Could you check a few things on this model? Use its own coordinates, in mm. Face numbers are marked on the shaded views. A direction names the side the tool comes from. Coordinates: 2 decimals unless noted, no trailing zeros. Loops run counter-clockwise (first coordinate to the right, second up) from the corner with the lowest first, then second, coordinate; pieces in that order, holes last. Notation, with made-up numbers: (-23.75, 7) -> (19.25, 7) arc R25 cw to (19.25, 42) -> close; hole circle Ø7 at (-10, 88). An arc over 180 degrees is marked (long way). One line per question, with ' | ' between items.
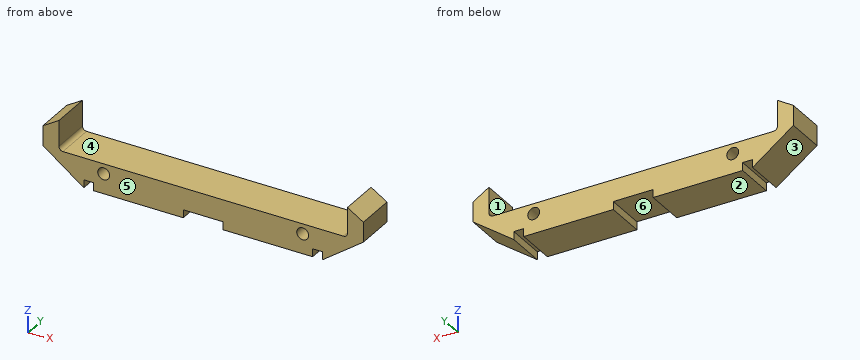
Autodesk Inventor part; units mm, degrees
ref_plane "YZ Plane" through (0, 0, 0) normal (1, 0, 0) x (0, 1, 0)
ref_plane "XZ Plane" through (0, 0, 0) normal (0, 1, 0) x (-1, 0, 0)
ref_plane "XY Plane" through (0, 0, 0) normal (0, 0, 1) x (1, 0, 0)
sketch "Esquisse1" plane through (0, 0, 0) normal (0, 1, 0) x (-1, 0, 0)
  circle A0 centre (0, 0) radius 25 construction
  line L0 (-25, 0) -> (25, 0) construction
  arc A1 (-75, -80.7775) -> (-75, 80.7775) centre (-25, 0) ccw construction
  arc A2 (75, 80.7775) -> (75, -80.7775) centre (25, 0) ccw construction
  line L1 (0, 25) -> (0, 0) construction
  line L2 (-75, 80.7775) -> (75, 80.7775)
  line L3 (-75, -80.7775) -> (75, -80.7775)
  arc A3 (75, -80.7775) -> (75, 80.7775) centre (25, 0) ccw
  arc A4 (-75, 80.7775) -> (-75, -80.7775) centre (-25, 0) ccw
  dimension "d0" = 50
  dimension "d1" = 190
  dimension "d2" = 150
extrude "Extrusion1" add sketch "Esquisse1" along normal mid plane 20
sketch "Esquisse4" plane through (0, -10, 0) normal (0, -1, 0) x (1, 0, 0)
  line L0 (-50, 40) -> (50, 40) construction
  line L1 (50, 40) -> (50, -40) construction
  line L2 (50, -40) -> (-50, -40) construction
  line L3 (-50, -40) -> (-50, 40) construction
  circle A0 centre (-50, 40) radius 3
  circle A1 centre (50, 40) radius 3
  circle A2 centre (50, -40) radius 3
  circle A3 centre (-50, -40) radius 3
  line L4 (75, 80.7775) -> (-75, 80.7775)
  point P0 (0, 0)
  dimension "d15" = 80
  dimension "d16" = 100
  dimension "d17" = 50
  dimension "d18" = 40
  dimension "d19" = 6
  dimension "d20" = 6
  dimension "d21" = 6
  dimension "d22" = 6
  dimension "d25" = 40.7775
extrude "Extrusion4" cut sketch "Esquisse4" against normal through all
sketch "Esquisse12" plane through (0, -10, 0) normal (0, -1, 0) x (1, 0, 0)
  circle A0 centre (50, -40) radius 3
  circle A1 centre (-50, 40) radius 3
  circle A2 centre (50, 40) radius 3
  circle A3 centre (-50, -40) radius 3
  line L0 (75, 80.7775) -> (-75, 80.7775)
  arc A4 (-75, 80.7775) -> (-75, -80.7775) centre (-25, 0) ccw
  line L1 (-75, -80.7775) -> (75, -80.7775)
  arc A5 (75, -80.7775) -> (75, 80.7775) centre (25, 0) ccw
  line L2 (-72.5, 60) -> (72.5, 60)
  line L3 (72.5, 60) -> (72.5, 45)
  line L4 (72.5, 45) -> (-72.5, 45)
  line L5 (-72.5, 45) -> (-72.5, 60)
  line L6 (-60, 45) -> (60, 45)
  line L7 (60, 45) -> (60, 30)
  line L8 (60, 30) -> (-60, 30)
  line L9 (-60, 30) -> (-60, 45)
  line L10 (-72.5, 45) -> (-80.5, 45)
  line L11 (-80.5, 45) -> (-80.5, 55)
  line L12 (-80.5, 55) -> (-72.5, 55)
  line L13 (-72.5, 55) -> (-72.5, 45)
  line L14 (72.5, 45) -> (80.5, 45)
  line L15 (80.5, 45) -> (80.5, 55)
  line L16 (80.5, 55) -> (72.5, 55)
  line L17 (72.5, 55) -> (72.5, 45)
  line L18 (-60, 30) -> (-80.5, 45)
  line L19 (60, 30) -> (80.5, 45)
  line L20 (-80.5, 55) -> (-72.5, 60)
  line L21 (-72.5, 55) -> (-72.5, 60)
  line L22 (80.5, 55) -> (72.5, 60)
  line L23 (72.5, 60) -> (72.5, 55)
  line L24 (-60, 30) -> (-55, 30)
  line L25 (-55, 30) -> (-55, 34)
  line L26 (-55, 34) -> (-60, 34)
  line L27 (-60, 34) -> (-60, 30)
  line L28 (60, 30) -> (55, 30)
  line L29 (55, 30) -> (55, 34)
  line L30 (55, 34) -> (60, 34)
  line L31 (60, 34) -> (60, 30)
  line L32 (10, 30) -> (-10, 30)
  line L33 (-10, 30) -> (-10, 34)
  line L34 (-10, 34) -> (10, 34)
  line L35 (10, 34) -> (10, 30)
  point P0 (0, 0)
  dimension "d101" = 145
  dimension "d102" = 15
  dimension "d103" = 40.7775
  dimension "d105" = 72.5
  dimension "d106" = 10
  dimension "d107" = 10
  dimension "d108" = 10
  dimension "d109" = 8
  dimension "d110" = 8
  dimension "d111" = 5
  dimension "d112" = 5
  dimension "d116" = 5
  dimension "d117" = 4
  dimension "d118" = 5
  dimension "d119" = 4
  dimension "d120" = 4
  dimension "d121" = 20
  dimension "d122" = 10
  dimension "d144" = 5
extrude "Extrusion9" cut sketch "Esquisse12" against normal through all contours A5 L1 A4 L0 | L2 L3 L4 L5 | L9 L26 L25 L8 | L8 L29 L30 L7 | L33 L34 L35 L8
fillet "Congé1" radius 2 2 edges at (72.5, 0, 45) (-72.5, 0, 45)
equation "\"d20\" = d19"
equation "\"d21\" = d19"
equation "\"d22\" = d19"
properties part number "base"
Q1. Please list where these lines run through material, in increasing order: L1, parallel to Z at x = -50, y = 5.25; L2, parallel to X at y = -8.75, z = 39; L3, parallel to Z at x = -21, y = -3.5. Write a range as [from, to].
Values follow:
L1: z = [30, 37], [43, 45] | L2: x = [-72.3, -52.83], [-47.17, 47.17], [52.83, 72.3] | L3: z = [30, 45]
Q2. Imagine slicing it at A-A on x = 50. Write out the boundary of the cut face in (y, z).
Values follow:
outline: (-10, 30) -> (10, 30) -> (10, 37) -> (-10, 37) -> close; (-10, 43) -> (10, 43) -> (10, 45) -> (-10, 45) -> close
Q3. We'd pull the mould along X, two halves only. Please class the marked faces 1, 2 and 3: released by +X, released by -X, zero draft, split by the parting line, or undercut.
Values follow:
face 1: undercut | face 2: zero draft | face 3: released by -X
Q4. Imagine slicing it at C-C on z = 40. Write out the boundary of the cut face in (x, y), plus the area to 3 significant figures.
Values follow:
outline: (-73.67, -10) -> (-53, -10) -> (-53, 10) -> (-73.67, 10) -> close; (-47, -10) -> (47, -10) -> (47, 10) -> (-47, 10) -> close; (53, -10) -> (73.67, -10) -> (73.67, 10) -> (53, 10) -> close | area: 2,710 mm2
Q5. For pin 1 (5 mm diameter, centred on y = -1, z = 38, fed in from -X); pin 2 (5.5 mm diameter, centred on x = -56.5, y = -1.5, fed in from -Z); pin 3 (2 mm diameter, centred on y = 3, z = 32, fed in from +X); pin 4 (3 mm diameter, centred on y = -3, z = 33, fed in from -X), each with a flat end and sliding along its axis, tell me the tip position at first contact or that it passes through.
Values follow:
pin 1: stops at x = -74.35 | pin 2: stops at z = 30 | pin 3: stops at x = 64.1 | pin 4: stops at x = -66.15
Q6. Imagine slicing it at D-D on z = 32. Write out the boundary of the cut face in (x, y), plus the area to 3 significant figures.
Values follow:
outline: (-62.73, -10) -> (-60, -10) -> (-60, 10) -> (-62.73, 10) -> close; (-55, -10) -> (-10, -10) -> (-10, 10) -> (-55, 10) -> close; (10, -10) -> (55, -10) -> (55, 10) -> (10, 10) -> close; (60, -10) -> (62.73, -10) -> (62.73, 10) -> (60, 10) -> close | area: 1,910 mm2
Q7. Imagine slicing it at B-B on y = 1. Write out the boundary of the cut face in (x, z), plus the area to 3 significant figures.
Values follow:
outline: (-80.5, 45) -> (-60, 30) -> (-60, 34) -> (-55, 34) -> (-55, 30) -> (-10, 30) -> (-10, 34) -> (10, 34) -> (10, 30) -> (55, 30) -> (55, 34) -> (60, 34) -> (60, 30) -> (80.5, 45) -> (80.5, 55) -> (72.5, 60) -> (72.5, 47) arc R2 cw to (70.5, 45) -> (-70.5, 45) arc R2 cw to (-72.5, 47) -> (-72.5, 60) -> (-80.5, 55) -> close; hole circle Ø6 at (-50, 40); hole circle Ø6 at (50, 40) | area: 2,130 mm2
Q8. For the marked faces 4, 5 and 6, which set-ups out of +Z, -Z, +X, -X, +Y, -Y let a thin tool reach every point of the face, with its end or its side?
Values follow:
face 4: +Z, +Y, -Y | face 5: +Z, -Z, +X, -X, -Y | face 6: -Z, +Y, -Y
